```python
from build123d import *

# Parameters (mm, degrees)
ESBO_O1_W                = 40
ESBO_O1_H                = 40
RESSALTO_EXTRUS_O1_DEPTH = 40
FILETE1_R                = 1
ESBO_O10_W               = 26
ESBO_O10_H               = 26
CORTE_EXTRUS_O3_DEPTH    = 7
ESBO_O11_W               = 26
ESBO_O11_H               = 26
CORTE_EXTRUS_O6_DEPTH    = 6
ESBO_O12_W               = 26
ESBO_O12_H               = 26
CORTE_EXTRUS_O7_DEPTH    = 6
ESBO_O13_W               = 26
ESBO_O13_H               = 26
CORTE_EXTRUS_O8_DEPTH    = 7


with BuildPart() as part:
    # Esboço1 → Ressalto-extrusão1 (new body)
    with BuildSketch(Plane(origin=(0, 0, 0), x_dir=(1, 0, 0), z_dir=(0, 1, 0))):
        with Locations((-13.703200382, -28.10068404)):
            Rectangle(ESBO_O1_W, ESBO_O1_H)
    extrude(amount=RESSALTO_EXTRUS_O1_DEPTH)

    # Loft de corte4: read off the stored shape, not the designer's step
    # Loft de corte4: loft between two sections, ruled curve by curve
    loft_de_corte4_from = [
        Edge.make_bspline([(-11.144198007, 40, 18.927950759), (7.201268555, 40, 24.04595551), (2.083263805, 40, 42.391422072), (-16.262202757, 40, 37.273417321), (-34.607669319, 40, 32.155412571), (-29.489664569, 40, 13.809946009), (-11.144198007, 40, 18.927950759)], [0, 0, 0, 0, 0.5, 0.5, 0.5, 1, 1, 1, 1], 3, [1, 0.333333333, 0.333333333, 1, 0.333333333, 0.333333333, 1]),
    ]
    loft_de_corte4_to = [
        Edge.make_bspline([(-10.380671839, 11.42, 27.000318611), (-8.179940979, 11.42, 33.645375697), (-14.824998066, 11.42, 35.846106557), (-17.025728925, 11.42, 29.20104947), (-19.226459785, 11.42, 22.555992384), (-12.581402699, 11.42, 20.355261524), (-10.380671839, 11.42, 27.000318611)], [0, 0, 0, 0, 0.5, 0.5, 0.5, 1, 1, 1, 1], 3, [1, 0.333333333, 0.333333333, 1, 0.333333333, 0.333333333, 1]),
    ]
    loft_de_corte4 = Solid(Shell([*[Face.make_surface_from_curves(loft_de_corte4_from[k], loft_de_corte4_to[k]) for k in range(1)], Face(Wire(loft_de_corte4_from)), Face(Wire(loft_de_corte4_to))]))
    add(loft_de_corte4, mode=Mode.SUBTRACT)

    # Filete1
    filete1_edges = [part.edges().sort_by_distance(p)[0] for p in [
        (-17.025728925, 11.42, 29.20104947),
    ]]
    fillet(filete1_edges, radius=FILETE1_R)

    # Esboço10 → Corte-extrusão3 (cut)
    with BuildSketch(Plane.ZY.offset(33.703200382)):
        with Locations((28.10068404, 20)):
            Rectangle(ESBO_O10_W, ESBO_O10_H)
    extrude(amount=-CORTE_EXTRUS_O3_DEPTH, mode=Mode.SUBTRACT)

    # Esboço11 → Corte-extrusão6 (cut)
    with BuildSketch(Plane(origin=(0, 0, 8.10068404), x_dir=(-1, 0, 0), z_dir=(0, 0, -1))):
        with Locations((13.703200382, 20)):
            Rectangle(ESBO_O11_W, ESBO_O11_H)
    extrude(amount=-CORTE_EXTRUS_O6_DEPTH, mode=Mode.SUBTRACT)

    # Esboço12 → Corte-extrusão7 (cut)
    with BuildSketch(Plane.XY.offset(48.10068404)):
        with Locations((-13.703200382, 20)):
            Rectangle(ESBO_O12_W, ESBO_O12_H)
    extrude(amount=-CORTE_EXTRUS_O7_DEPTH, mode=Mode.SUBTRACT)

    # Esboço13 → Corte-extrusão8 (cut)
    with BuildSketch(Plane(origin=(6.296799618, 0, 0), x_dir=(0, 0, -1), z_dir=(1, 0, 0))):
        with Locations((-28.10068404, 20)):
            Rectangle(ESBO_O13_W, ESBO_O13_H)
    extrude(amount=-CORTE_EXTRUS_O8_DEPTH, mode=Mode.SUBTRACT)


solid = part.part
```
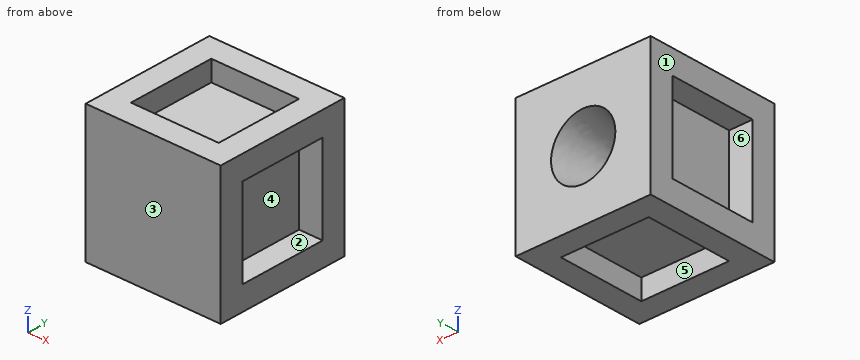
Part model, mm, in its own coordinate system. Face numbers are marked on the shaded views. A direction names the side the tool comes from. Round coordinates to 2 decimals unless told otherwise and drop trailing zeros. Write each loop counter-clockwise with the first axis right and the second up, starting at its lowest first coordinate (ties: lowest second). Pieces come first, ordered by that corner, then holes.
Item 1: Probe L1, parallel to Z at x = 1, y = 21; L2, parallel to Y at x = -7, z = 44; L3, parallel to X at y = 20, z = 42.5. List the from-to ranges inside material, lowest first.
Results:
L1: z = 8.1 to 15.1, 41.1 to 48.1
L2: y = 0 to 7, 33 to 40
L3: x = -33.7 to -26.7, -0.7 to 6.3
Item 2: Two-plate mould, pull along Y, no slides. Class the marked faces 1, 2 and 3: +Y half, -Y half, draft (parallel to the pull), parting line (faces both ways), or undercut.
Results:
face 1: draft
face 2: undercut
face 3: -Y half
Item 3: Cut at D-D, the plane y = 8. Give the cut face in (x, z).
Results:
outline: (-33.7, 8.1) - (-26.7, 8.1) - (-26.7, 14.1) - (-0.7, 14.1) - (-0.7, 8.1) - (6.3, 8.1) - (6.3, 15.1) - (-0.7, 15.1) - (-0.7, 41.1) - (6.3, 41.1) - (6.3, 48.1) - (-0.7, 48.1) - (-0.7, 42.1) - (-26.7, 42.1) - (-26.7, 48.1) - (-33.7, 48.1) - (-33.7, 41.1) - (-26.7, 41.1) - (-26.7, 15.1) - (-33.7, 15.1) - close
Item 4: Cut at A-A, the plane x = -28. Give the cut face in (y, z).
Results:
outline: (0, 8.1) - (40, 8.1) - (40, 48.1) - (0, 48.1) - close; hole (7, 15.1) - (33, 15.1) - (33, 41.1) - (7, 41.1) - close
Item 5: Drop flat-ended pins along their axis: pin 1 Ø7.5 at (x, z) = (-31, 27.5) entering from -Y; pin 2 Ø13 at (x, y) = (-18.5, 19.5) entering from -Z; pin 3 Ø13 at (y, z) = (24, 27) entering from +X; pin 4 Ø3 at (x, y) = (-5, 16.5) entering from +Z. Give the stop position or say it passes through.
Results:
pin 1: stops at y = 0
pin 2: stops at z = 14.1
pin 3: stops at x = -0.7
pin 4: stops at z = 42.1
Item 6: Cut at C-C, the plane z = 44. Give the cut face in (x, y).
Results:
outline: (-33.7, 0) - (6.3, 0) - (6.3, 40) - (-33.7, 40) - close; hole (-26.7, 7) - (-0.7, 7) - (-0.7, 33) - (-26.7, 33) - close
Item 7: Cut at B-B, the plane z = 17.5. Give the cut face in (x, y).
Results:
outline: (-33.7, 0) - (6.3, 0) - (6.3, 7) - (-0.7, 7) - (-0.7, 33) - (6.3, 33) - (6.3, 40) - (-33.7, 40) - (-33.7, 33) - (-26.7, 33) - (-26.7, 7) - (-33.7, 7) - close
Item 8: Which spindle directions (+Z, -Z, +X, -X, +Y, -Y) get a long thin tool onto all of the face, cutting with end or side? Do the marked faces 4, 5 and 6. Say none if no direction does.
Results:
face 4: +X
face 5: -Z
face 6: -X
